from build123d import *

# Parameters (mm, degrees)
BOSS_EXTRU_1_DEPTH           = 10
ENL_V_MAT_EXTRU_1_DEPTH      = 11
R_P_TITION_CIRCULAIRE1_COUNT = 10
R_P_TITION_CIRCULAIRE1_ANGLE = 73.8
R_P_TITION_CIRCULAIRE2_COUNT = 10
R_P_TITION_CIRCULAIRE2_ANGLE = 73.8


with BuildPart() as part:
    # Esquisse1 → Boss.-Extru.1 (new body)
    with BuildSketch(Plane.XY):
        with BuildLine():
            Line((-140.132008959, 22.5), (-106.879003857, 22.5))
            ThreePointArc((-106.879003857, 22.5), (58.598335981, 167), (224.07567582, 22.5))
            Line((224.07567582, 22.5), (257.328680921, 22.5))
            ThreePointArc((257.328680921, 22.5), (58.598335981, 200), (-140.132008959, 22.5))
        make_face()
    extrude(amount=BOSS_EXTRU_1_DEPTH)

    # Esquisse2 → Enlèv. mat.-Extru.1 (cut, through all)
    with BuildSketch(Plane.XY.offset(10)):
        with BuildLine():
            Line((50.098335981, 179.5), (50.098335981, 186.5))
            ThreePointArc((50.098335981, 186.5), (58.598335981, 195), (67.098335981, 186.5))
            Line((67.098335981, 186.5), (67.098335981, 179.5))
            ThreePointArc((67.098335981, 179.5), (58.598335981, 171), (50.098335981, 179.5))
        make_face()
    enl_v_mat_extru_1 = extrude(amount=-ENL_V_MAT_EXTRU_1_DEPTH, mode=Mode.SUBTRACT)

    # Répétition circulaire1: Enlèv. mat.-Extru.1 ×10 about axis
    r_p_tition_circulaire1_axis = Axis((58.598335981, 0, 0), (0, 0, -1))
    for i in range(1, R_P_TITION_CIRCULAIRE1_COUNT):
        add(enl_v_mat_extru_1.rotate(r_p_tition_circulaire1_axis, i * R_P_TITION_CIRCULAIRE1_ANGLE / (R_P_TITION_CIRCULAIRE1_COUNT - 1)), mode=Mode.SUBTRACT)

    # Répétition circulaire2: Enlèv. mat.-Extru.1 ×10 about axis
    r_p_tition_circulaire2_axis = Axis((58.598335981, 0, 0), (0, 0, 1))
    for i in range(1, R_P_TITION_CIRCULAIRE2_COUNT):
        add(enl_v_mat_extru_1.rotate(r_p_tition_circulaire2_axis, i * R_P_TITION_CIRCULAIRE2_ANGLE / (R_P_TITION_CIRCULAIRE2_COUNT - 1)), mode=Mode.SUBTRACT)


solid = part.part
Can you work these out from the model? Positions are in its coordinate system, mm. A direction names the side the tool comes from. Coordinates: 2 decimals unless noted, no trailing zeros. Return JSON: item names as keys, results as strings. Group by question number.
Item 1: On a 3-axis mill with a long thin cutter (end or side, diameter ignored), from which of +Z, -Z, +X, -X, +Y, -Y can I reach the whole of each face in a straight line? I mean faces 4 (the flat face through (40.9, 182.4, 5.1)), 5 (the flat face through (-124, 22.5, 5)). Say none if no direction works.
Item 2: I'm going to push flat-ended pins straight in: pin 1 Ø5 at (x, z) = (124, 4.5) entering from +Y; pin 2 Ø3 at (x, z) = (-17.5, 8.5) entering from +Y; pin 3 Ø6 at (y, z) = (180, 5) entering from -X. Where does each tip first touch, or does it pass through?
Item 3: Imagine slicing it at A-A (z = 5.25). Give the number of separate pieces and of enclosed holes in the cut face, and give its area (3 significant figures).
Item 4: Thinking about a two-plate mould opening in X: for faces 1 (the flat face through (67.098, 183, 5)), 2 (the flat face through (57.7, 170.8, 0)), 3 (the flat face through (118.435, 173.202, 5.07)), which applies, released by +X, released by -X, zero draft, split by the parting line, or undercut?
Item 5: If I drill on L1, parallel to Y at x = 202, z = 5.5; L2, parallel to X at y = 154, z = 8.25; L3, parallel to X at y = 66.5, z = 0.5, over which ranges is the centre line in solid material (lowest first)? Write a range as from..to.
Verdict:
{
 "1": {"face 4": "+Z, -Z", "face 5": "+Z, -Z, +X, -X, -Y"},
 "2": {"pin 1": "stops at y = 189.85", "pin 2": "stops at y = 185.57", "pin 3": "stops at x = -34.52"},
 "3": {"separate pieces": "1", "enclosed holes": "19", "area": "11,000 mm^2"},
 "4": {"face 1": "undercut", "face 2": "zero draft", "face 3": "undercut"},
 "5": {"L1": "y = 85.59..93.37, 100.04..112.55, 130.07..139.41", "L2": "x = -69.01..-50.47, -30.73..-6, 123.2..147.93, 167.66..186.21", "L3": "x = -130.02..-108.58, -101.17..-94.59, 211.79..218.37, 225.77..247.22"}
}
